Part model, mm, in its own coordinate system. Give positions to 0.01 mm unless a question says otherwise; leave off trailing zeros. Order: outer loops, then holes, each group sorted by start corner. A loop starts at its lowest first (then second) coordinate and runs counter-clockwise, first axis right, second up. Notation, with made-up numbers: M 72.25,73.5 L 126.25,73.5 A12 cw 126.25,86.5 Z; hole C 0.5,-9.75 d3. An arc over 180 degrees is marked long. Return JSON: item names as keys, results as strings.
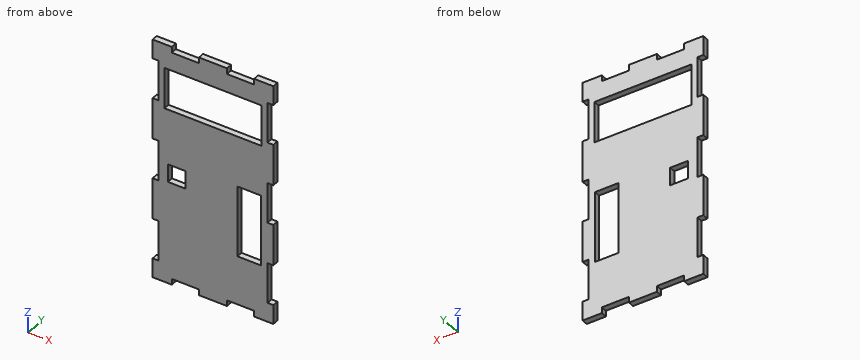
from build123d import *

# Parameters (mm, degrees)
F0_W     = 63.5
F0_H     = 127
F0_W_2   = 9.398
F0_H_2   = 9.398
F0_W_3   = 12.4
F0_H_3   = 37.3
F0_W_4   = 51.054
F0_H_4   = 21.59
F1_DEPTH = 3.175
F2_W     = 14.3
F2_H     = 3.075
F2_W_2   = 3.075
F2_H_2   = 21.2
F3_DEPTH = 25


# Not quite as in the source:
# - a feature of the source that left no trace in its solid (it failed there, or was rolled back) is left out
# - a length typed as a fraction of an inch, garbled in the dataset ("3 / 203.2 mm" for 3/8 in), is restored


with BuildPart() as f1:
    # F0 (on Front) → F1 (new body)
    with BuildSketch(Plane.XZ):
        Rectangle(F0_W, F0_H)
        with Locations((-19.05, -4.699)):
            Rectangle(F0_W_2, F0_H_2, mode=Mode.SUBTRACT)
        with Locations((19.05, -16.11)):
            Rectangle(F0_W_3, F0_H_3, mode=Mode.SUBTRACT)
        with Locations((0, 40.005)):
            Rectangle(F0_W_4, F0_H_4, mode=Mode.SUBTRACT)
    extrude(amount=-F1_DEPTH)

    # F2 (on face) → F3 (cut)
    with BuildSketch(Plane(origin=(0, 3.175, 0), x_dir=(-1, 0, 0), z_dir=(0, 1, 0))):
        with Locations((14.5, 61.9625)):
            Rectangle(F2_W, F2_H)
        with Locations((-14.5, 61.9625)):
            Rectangle(F2_W, F2_H)
        with Locations((-30.2125, -42.8)):
            Rectangle(F2_W_2, F2_H_2)
        with Locations((-30.2125, 0)):
            Rectangle(F2_W_2, F2_H_2)
        with Locations((-30.2125, 42.8)):
            Rectangle(F2_W_2, F2_H_2)
        with Locations((30.2125, -42.8)):
            Rectangle(F2_W_2, F2_H_2)
        with Locations((30.2125, 0)):
            Rectangle(F2_W_2, F2_H_2)
        with Locations((30.2125, 42.8)):
            Rectangle(F2_W_2, F2_H_2)
        with Locations((-14.5, -61.9625)):
            Rectangle(F2_W, F2_H)
        with Locations((14.5, -61.9625)):
            Rectangle(F2_W, F2_H)
    extrude(amount=-F3_DEPTH, mode=Mode.SUBTRACT)


solid = f1.part
Q1. Band-saw the part on B-B (x = 15.5). Give the cut face in (y, z) (3 decimals), then the cut area to 3 significant figures.
Established:
{"outline": "M 0,-60.425 L 3.175,-60.425 L 3.175,-34.76 L 0,-34.76 Z; M 0,2.54 L 3.175,2.54 L 3.175,29.21 L 0,29.21 Z; M 0,50.8 L 3.175,50.8 L 3.175,60.425 L 0,60.425 Z", "area": "197 mm²"}
Q2. Band-saw the part on D-D (z = -2). Give the cut face in (x, y) (3 decimals), then the cut area to 3 significant figures.
Established:
{"outline": "M -28.675,0 L -23.749,0 L -23.749,3.175 L -28.675,3.175 Z; M -14.351,0 L 12.85,0 L 12.85,3.175 L -14.351,3.175 Z; M 25.25,0 L 28.675,0 L 28.675,3.175 L 25.25,3.175 Z", "area": "113 mm²"}
Q3. Pin check, flat tip, straight feed: pin 1 (1.6 mm diameter, centred on y = 1.5, z = -4, fed in from +X) (3 decimals). Stop position of the tip, or through.
Established:
{"pin 1": "stops at x = 28.675"}
Q4. Band-saw the part on A-A (x = -2). Give the cut face in (y, z) (3 decimals).
Established:
{"outline": "M 0,-63.5 L 3.175,-63.5 L 3.175,29.21 L 0,29.21 Z; M 0,50.8 L 3.175,50.8 L 3.175,63.5 L 0,63.5 Z"}
Q5. Probe line 1 along Z through (x, y) = (17.5, 2.4) (3 decimals); line 2 along Z through (x, y) = (-21, 2.3) (3 decimals); line 3 along Z through (x, y) = (29, 1.55). List the from-to ranges inside material, lowest first.
Established:
{"line 1": "z = -60.425 to -34.76, 2.54 to 29.21, 50.8 to 60.425", "line 2": "z = -60.425 to -9.398, 0 to 29.21, 50.8 to 60.425", "line 3": "z = -63.5 to -53.4, -32.2 to -10.6, 10.6 to 32.2, 53.4 to 63.5"}
Q6. Band-saw the part on C-C (z = 34). Give the cut face in (x, y) (3 decimals).
Established:
{"outline": "M -28.675,0 L -25.527,0 L -25.527,3.175 L -28.675,3.175 Z; M 25.527,0 L 28.675,0 L 28.675,3.175 L 25.527,3.175 Z"}
